CAD build for the part. Positions are in the model's coordinates, mm. A direction names the side the tool comes from. Give positions to 0.01 mm unless a question says otherwise; leave off trailing zeros. Order: outer loops, then holes, each group sorted by start corner. A loop starts at its lowest first (then second) coordinate and runs counter-clockwise, first axis right, second up.
Item 1: Band-saw the part on B-B on y = 6.75. Give the cut face in (x, z), plus the area to 3 significant figures.
Item 2: Which spindle directions (+Z, -Z, +X, -X, +Y, -Y) get a long thin tool onto all of the face, cutting with end or side? Do faces 1 (the flat face through (-3, 3, 4)), 2 (the cylindrical face through (-9, 2, 2)), 3 (the flat face through (0, 9, 0)), 4 (the flat face through (3, 3, 4)), 5 (the flat face through (0, 6.5, 5)). Say none if no direction does.
Item 3: Two-plate mould, pull along Y, no slides. Class faces 6 (the cylindrical face through (-0.22, 17.248, 1.479)), 7 (the cylindrical face through (0, 16, 1)), 8 (the flat face through (-10, 6, 1)): released by +Y, released by -Y, zero draft, split by the parting line, or undercut.
Item 4: Band-saw the part on D-D on x = 4.6. Give the cut face in (y, z).
Item 5: Wall check: L1, parallel to X at y = 6.75, z = 1.45; L2, parallel to Y at x = 0, z = 1.45; L3, parallel to Z at x = -5.5, y = 5.5. Give the ranges that are in metal, low to high.
Item 6: Band-saw the part on A-A on x = 0. Give the cut face in (y, z).
Item 7: Band-saw the part on C-C on y = 14.5. Give the cut face in (x, z).
Item 8: Flat gauge pins, fed straight in: P1, Ø1, axis at x = -3.5, z = 7, coming from the -Y side; P2, Ø4, axis at x = 2.5, y = 4.5, coming from the +Z side; P3, Ø1, axis at y = 6, z = 5.5, coming from the -X side. Where does each tip first touch, or does it go through?
Autodesk Inventor part; units mm, degrees
ref_plane "YZ Plane" through (0, 0, 0) normal (1, 0, 0) x (0, 1, 0)
ref_plane "XZ Plane" through (0, 0, 0) normal (0, 1, 0) x (-1, 0, 0)
ref_plane "XY Plane" through (0, 0, 0) normal (0, 0, 1) x (1, 0, 0)
sketch "Esquisse1" plane through (0, 0, 0) normal (0, 0, 1) x (1, 0, 0)
  arc A0 (10, 7.25) -> (-10, 7.25) centre (0, 7.25) ccw
  line L0 (-10, 0) -> (10, 0)
  line L1 (10, 0) -> (10, 7.25)
  line L2 (-10, 7.25) -> (-10, 0)
  point P0 (0, 0)
  point P1 (0, 4.9938)
  point P2 (0, 0)
  dimension "d0" = 20
  dimension "d1" = 17.25
extrude "Extrusion1" add sketch "Esquisse1" along normal blind 3
fillet "Congé1" radius 5 2 edges at (-10, 0, 1.5) (10, 0, 1.5)
sketch "Esquisse2" plane through (-5, 0, 0) normal (0, -1, 0) x (1, 0, 0)
  line L0 (2, 3) -> (8, 3)
  line L1 (8, 3) -> (8, 5)
  line L2 (5, 8) -> (5, 8)
  line L3 (2, 5) -> (2, 3)
  line L4 (0, 0) -> (10, 0)
  line L5 (0, 3) -> (10, 3)
  arc A0 (5, 8) -> (2, 5) centre (5, 5) ccw
  arc A1 (8, 5) -> (5, 8) centre (5, 5) ccw
  point P0 (5, 0)
  point P1 (5, 3)
  point P2 (5, 0)
  dimension "d5" = 8
  dimension "d7" = 3
  dimension "d8" = 6
extrude "Extrusion2" add sketch "Esquisse2" against normal blind 6.5
sketch "Esquisse3" plane through (0, 0, 3) normal (0, 0, 1) x (1, 0, 0)
  line L0 (-3, 0) -> (3, 0)
  point P0 (0, 0)
  point P1 (-4.6, 6.75)
  point P2 (4.6, 6.75)
  point P3 (0, 14.5)
  point P4 (0, 0)
  dimension "d11" = 9.2
  dimension "d12" = 4.6
  dimension "d13" = 6.75
  dimension "d14" = 14.5
hole "Perçage1" at (-4.6, 6.75, 3) at (4.6, 6.75, 3) at (0, 14.5, 3) direction (0, 0, -1) diameter 3 depth 8 tip angle 118
equation "\"d7\" = 0.5 * d8"
properties part number "Support capteur" material "Plastique ABS"
The answers:
1. outline: (-10, 0) - (-6.1, 0) - (-6.1, 3) - (-10, 3) - close; (-3.1, 0) - (3.1, 0) - (3.1, 3) - (-3.1, 3) - close; (6.1, 0) - (10, 0) - (10, 3) - (6.1, 3) - close
1. area: 42.0 mm2
2. face 1: +Z, -X, +Y, -Y
2. face 2: +Z, -Z, -X, -Y
2. face 3: -Z, +X, -X, +Y, -Y
2. face 4: +Z, +X, +Y, -Y
2. face 5: +Z, +X, -X, +Y
3. face 6: released by +Y
3. face 7: undercut
3. face 8: zero draft
4. outline: (0, 0) - (5.25, 0) - (5.25, 3) - (0, 3) - close; (8.25, 0) - (16.13, 0) - (16.13, 3) - (8.25, 3) - close
5. L1: x = -10 to -6.1, -3.1 to 3.1, 6.1 to 10
5. L2: y = 0 to 13, 16 to 17.25
5. L3: z = 0 to 3
6. outline: (0, 0) - (13, 0) - (13, 3) - (6.5, 3) - (6.5, 8) - (0, 8) - close; (16, 0) - (17.25, 0) - (17.25, 3) - (16, 3) - close
7. outline: (-6.89, 0) - (-1.5, 0) - (-1.5, 3) - (-6.89, 3) - close; (1.5, 0) - (6.89, 0) - (6.89, 3) - (1.5, 3) - close
8. P1: passes through
8. P2: stops at z = 7.96
8. P3: stops at x = -3
